```python
from build123d import *

# Parameters (mm, degrees)
SKETCH1_R               = 20
SKETCH1_R_2             = 12.6
BOSS_EXTRUDE1_DEPTH     = 70
SKETCH2_R               = 1.5
CUT_EXTRUDE1_DEPTH      = 10
SKETCH3_R               = 1.55
CUT_EXTRUDE2_DEPTH      = 21
CUT_EXTRUDE2_DEPTH_BACK = 21


with BuildPart() as part:
    # Sketch1 → Boss-Extrude1 (new body)
    with BuildSketch(Plane.XY):
        Circle(SKETCH1_R)
        Circle(SKETCH1_R_2, mode=Mode.SUBTRACT)
    extrude(amount=BOSS_EXTRUDE1_DEPTH)

    # Sketch2 → Cut-Extrude1 (cut)
    with BuildSketch(Plane(origin=(0, 0, 0), x_dir=(-1, 0, 0), z_dir=(0, 0, -1))):
        with Locations((0, 15.25)):
            Circle(SKETCH2_R)
        with Locations((15.25, 0)):
            Circle(SKETCH2_R)
        with Locations((0, -15.25)):
            Circle(SKETCH2_R)
        with Locations((-15.25, 0)):
            Circle(SKETCH2_R)
    extrude(amount=-CUT_EXTRUDE1_DEPTH, mode=Mode.SUBTRACT)

    # Sketch3 → Cut-Extrude2 (cut, two sides)
    with BuildSketch(Plane(origin=(0, 0, 0), x_dir=(0, 0, -1), z_dir=(1, 0, 0))) as cut_extrude2_sk:
        with Locations((-45.5, 0)):
            Circle(SKETCH3_R)
        with Locations((-24.5, 0)):
            Circle(SKETCH3_R)
    extrude(amount=CUT_EXTRUDE2_DEPTH, mode=Mode.SUBTRACT)
    extrude(cut_extrude2_sk.sketch, amount=-CUT_EXTRUDE2_DEPTH_BACK, mode=Mode.SUBTRACT)


solid = part.part
```
Here's how the part is built. I have some questions about the finished solid (model axes, mm). A direction names the side the tool comes from. Coordinates: 2 decimals unless noted, no trailing zeros. Loops run counter-clockwise (first coordinate to the right, second up) from the corner with the lowest first, then second, coordinate; pieces in that order, holes last. Notation, with made-up numbers: (-38, 10.25) - (9, 10.25) arc R15 cw to (9, 17.25) - close; hole circle Ø4 at (48, -17). An arc over 180 degrees is marked (long way). Return JSON: item names as keys, results as strings. Group by question number.
Item 1: If we section it at A-A on x = 0: Write out the boundary of the cut face in (y, z).
Item 2: If we section it at D-D on y = -8: Write out the boundary of the cut face in (x, z), and give its area (3 significant figures).
Item 3: If we section it at B-B on y = 0: State how many separate pieces and enclosed holes the cut face has, and give its area (3 significant figures).
Item 4: On a 3-axis mill with a long thin cutter (end or side, diameter ignored), from which of +Z, -Z, +X, -X, +Y, -Y can I reach the whole of each face in a straight line? I mean faces 4 (the face through (-13.75, 0.07, 4.93)), 5 (the face through (-9.999, -7.667, 34.51)). Say none if no direction works.
Item 5: If we section it at C-C on z = 45.5: Write out the boundary of the cut face in (x, y), and give its area (3 significant figures).
Item 6: Will these pins go through, and if not, where does the flat tip stop? P1, Ø5, axis at y = 13.5, z = 11.5, coming from the +X side; P2, Ø6, axis at x = 7.5, z = 27, coming from the -Y side; P3, Ø6, axis at x = 12, z = 39.5, coming from the -Y side.
Item 7: We'd pull the mould along X, two halves only. Please class faces 1 (the face through (16.2, -0.594, 23.068)), 2 (the face through (-15, 0, 10)), 3 (the face through (-4.336, -19.524, 34.51)): +X half, -X half, draft (parallel to the pull), parting line (faces both ways), or undercut.
Item 8: I need wall thicknesses on line 1 (Y direction, x = 0, z = 6.25); line 2 (Z direction, x = 18.25, y = 0); line 3 (Z direction, x = -15, y = -1). Which ranges of each line are inside material? Lowest first, please. Write a range as from..to.
Calculated:
{
 "1": {"outline": "(-20, 0) - (-16.75, 0) - (-16.75, 10) - (-13.75, 10) - (-13.75, 0) - (-12.6, 0) - (-12.6, 70) - (-20, 70) - close; (12.6, 0) - (13.75, 0) - (13.75, 10) - (16.75, 10) - (16.75, 0) - (20, 0) - (20, 70) - (12.6, 70) - close"},
 "2": {"outline": "(-18.33, 0) - (-9.73, 0) - (-9.73, 70) - (-18.33, 70) - close; (9.73, 0) - (18.33, 0) - (18.33, 70) - (9.73, 70) - close", "area": "1,200 mm^2"},
 "3": {"separate pieces": "6", "enclosed holes": "0", "area": "884 mm^2"},
 "4": {"face 4": "-Z", "face 5": "+Z, -Z"},
 "5": {"outline": "(-19.94, -1.55) arc R20 ccw to (19.94, -1.55) - (12.5, -1.55) arc R12.6 cw to (-12.5, -1.55) - close; (-19.94, 1.55) - (-12.5, 1.55) arc R12.6 cw to (12.5, 1.55) - (19.94, 1.55) arc R20 ccw to start", "area": "712 mm^2"},
 "6": {"P1": "stops at x = 16.7", "P2": "stops at y = -19.49", "P3": "stops at y = -17.86"},
 "7": {"face 1": "draft", "face 2": "undercut", "face 3": "parting line"},
 "8": {"line 1": "y = -20..-16.75, -13.75..-12.6, 12.6..13.75, 16.75..20", "line 2": "z = 0..22.95, 26.05..43.95, 47.05..70", "line 3": "z = 10..23.32, 25.68..44.32, 46.68..70"}
}
